from build123d import *

# Parameters (mm, degrees)
SKETCH2_R          = 1.65
CUT_EXTRUDE1_DEPTH = 10


with BuildPart() as part:
    # Sketch1 → Revolve1 (revolve)
    with BuildSketch(Plane.XY):
        Polygon((0, 2.2), (6.9, 2.2), (6.9, 0), (8.1, 0), (8.1, 2.8), (9.7, 2.8), (9.7, 3.8), (8, 5), (0, 5), align=None)
    revolve(axis=Axis((0, 0, 0), (0, 1, 0)))

    # Sketch2 → Cut-Extrude1 (cut)
    with BuildSketch(Plane(origin=(0, 5, 0), x_dir=(1, 0, 0), z_dir=(0, 1, 0))):
        Circle(SKETCH2_R)
    extrude(amount=-CUT_EXTRUDE1_DEPTH, mode=Mode.SUBTRACT)


solid = part.part
Build history of the part. All positions in model axes, mm. A direction names the side the tool comes from. Round coordinates to 2 decimals unless told otherwise and drop trailing zeros. Write each loop counter-clockwise with the first axis right and the second up, starting at its lowest first coordinate (ties: lowest second). Pieces come first, ordered by that corner, then holes. Notation, with made-up numbers: (20, -33.5) - (70, -33.5) arc R22 ccw to (70, -15.5) - close; hole circle Ø5 at (21.25, -0.5). An arc over 180 degrees is marked (long way). One line per question, with ' | ' between items.
1. Band-saw the part on B-B, the plane z = 0. Write the cut outline in (x, y).
Results are:
outline: (-9.7, 2.8) - (-8.1, 2.8) - (-8.1, 0) - (-6.9, 0) - (-6.9, 2.2) - (-1.65, 2.2) - (-1.65, 5) - (-8, 5) - (-9.7, 3.8) - close; (1.65, 2.2) - (6.9, 2.2) - (6.9, 0) - (8.1, 0) - (8.1, 2.8) - (9.7, 2.8) - (9.7, 3.8) - (8, 5) - (1.65, 5) - close
2. Band-saw the part on C-C, the plane y = 2.5. Write the cut outline in (x, z).
Results are:
outline: circle Ø16.2 at (0, 0); hole circle Ø3.3 at (0, 0)
3. Band-saw the part on D-D, the plane y = 0.6. Write the cut outline in (x, z).
Results are:
outline: circle Ø16.2 at (0, 0); hole circle Ø13.8 at (0, 0)
4. Drop flat-ended pins along their axis: pin 1 Ø3 at (x, y) = (-5, 3) entering from -Z; pin 2 Ø4 at (x, z) = (-3.5, -1) entering from -Y; pin 3 Ø3 at (x, y) = (-7.5, 1.5) entering from +Z. Give the stop position or say it passes through.
Results are:
pin 1: z = -9.05 | pin 2: y = 2.2 | pin 3: z = 6.96
5. Mould opens along X. For faces 1 (the face through (0, 5, 2)), 2 (the face through (-0.9, 1.08, -6.84)), 3 (the face through (-1.756, 1.42, 7.907)) say: released by +X, released by -X, zero draft, split by the parting line, or undercut.
Results are:
face 1: zero draft | face 2: undercut | face 3: split by the parting line
6. Tool access for faces 4 (the face through (6, 2.8, 6)), 5 (the face through (-1.216, 3.62, -1.115)): list every direction of +Z, -Z, +X, -X, +Y, -Y with a clear straight run to the whole face (end or side of a thin tool).
Results are:
face 4: -Y | face 5: +Y, -Y
7. Band-saw the part on A-A, the plane x = 0. Write the cut outline in (y, z).
Results are:
outline: (0, -8.1) - (2.8, -8.1) - (2.8, -9.7) - (3.8, -9.7) - (5, -8) - (5, -1.65) - (2.2, -1.65) - (2.2, -6.9) - (0, -6.9) - close; (0, 6.9) - (2.2, 6.9) - (2.2, 1.65) - (5, 1.65) - (5, 8) - (3.8, 9.7) - (2.8, 9.7) - (2.8, 8.1) - (0, 8.1) - close
8. Drill centre lines: line 1 along Z through (x, y) = (0, 0.8); line 2 along Z through (x, y) = (0, 3.25); line 3 along Y through (x, z) = (5.5, 1). Where is each one in solid material? Low to high. Write a range as from..to.
Results are:
line 1: -8.1..-6.9, 6.9..8.1 | line 2: -9.7..-1.65, 1.65..9.7 | line 3: 2.2..5
